The model under review builds one solid part; all positions refer to its coordinate system, in mm. A direction names the side the tool comes from. Coordinates: 2 decimals unless noted, no trailing zeros. Write each loop counter-clockwise with the first axis right and the second up, starting at its lowest first coordinate (ties: lowest second). Pieces come first, ordered by that corner, then holes. Notation, with made-up numbers: (74, 25) -> (127, 25) arc R31 cw to (127, 50) -> close; hole circle Ø10 at (18, 26). An arc over 180 degrees is marked (long way). Write each question's results on one line, items separated by ' | '.
Autodesk Inventor part; units mm, degrees
ref_plane "Work Plane2" through (-3.9, 5.05, 12.4) normal (0, 0, 1) x (1, 0, 0)
ref_plane "Work Plane3" through (-3.9, 5.05, 8) normal (0, 0, 1) x (1, 0, 0)
ref_plane "Work Plane4" through (-13.9917, -57.9, 3) normal (0, 0, 1) x (1, 0, 0)
ref_plane "Work Plane1" through (0, 0, 0) normal (0, 0, 1) x (1, 0, 0)
sketch "Sketch1" plane through (0, 0, 0) normal (0, 0, 1) x (1, 0, 0)
  circle A0 centre (0, -8.95) radius 4.2
  circle A1 centre (0, 8.95) radius 4.2
  circle A2 centre (0, 0) radius 1.4
  circle A3 centre (3.9, 0) radius 0.1
  line L0 (8.9, 16.9) -> (7.9, 17.9)
  line L1 (7.9, 17.9) -> (-7.9, 17.9)
  line L2 (-7.9, 17.9) -> (-8.9, 16.9)
  line L3 (-8.9, 16.9) -> (-8.9, -16.9)
  line L4 (-8.9, -16.9) -> (-7.9, -17.9)
  line L5 (-7.9, -17.9) -> (7.9, -17.9)
  line L6 (7.9, -17.9) -> (8.9, -16.9)
  line L7 (8.9, -16.9) -> (8.9, 16.9)
  point P0 (0, 0)
ref_plane "Work Plane2" through (-3.9, 5.05, 12.4) normal (0, 0, 1) x (1, 0, 0)
ref_plane "Work Plane3" through (-3.9, 5.05, 8) normal (0, 0, 1) x (1, 0, 0)
extrude "Extrusion1" add sketch "Sketch1" along normal up to surface (8 mm away) contours A0 | A1 | L7 L6 L5 L4 L3 L2 L1 L0
sketch "Sketch2" plane through (-7.9, 17.9, 8) normal (0, 0, 1) x (1, 0, 0)
  line L0 (16.8, -1) -> (16.8, -34.8)
  line L1 (15.8, 0) -> (16.8, -1)
  line L2 (0, 0) -> (15.8, 0)
  line L3 (-1, -1) -> (0, 0)
  line L4 (-1, -34.8) -> (-1, -1)
  line L5 (0, -35.8) -> (-1, -34.8)
  line L6 (15.8, -35.8) -> (0, -35.8)
  line L7 (16.8, -34.8) -> (15.8, -35.8)
  circle A0 centre (11.8, -17.9) radius 0.1
  circle A1 centre (7.9, -17.9) radius 1.4
  point P0 (7.9, -17.9)
  point P1 (13.4, -17.9)
  point P2 (2.4, -17.9)
  dimension "d2" = 5.5
  dimension "d3" = 5.5
hole "Hole1" at (5.5, 0, 8) at (-5.5, 0, 8) direction (0, 0, -1) diameter 2.9 end through all counterbore diameter 6 counterbore depth 3.5
sketch "Sketch3" plane through (0, 0, 0) normal (0, 0, -1) x (-1, 0, 0)
  circle A0 centre (0, 8.95) radius 3.9 construction
  circle A1 centre (0, -8.95) radius 3.9 construction
  circle A2 centre (0, 8.95) radius 3.375
  circle A3 centre (0, -8.95) radius 3.375
  point P0 (0, 0)
  dimension "d11" = 6.75
  dimension "d12" = 6.75
extrude "Extrusion2" cut sketch "Sketch3" against normal blind 10
sketch "Sketch4" plane through (0, 0, 0) normal (0, 0, -1) x (-1, 0, 0)
  circle A0 centre (0, 8.95) radius 3.375
  circle A1 centre (0, -8.95) radius 3.375
  circle A2 centre (0, 8.95) radius 3.9
  circle A3 centre (0, -8.95) radius 3.9
  point P0 (0, 0)
  dimension "d15" = 7.8
  dimension "d16" = 7.8
extrude "Extrusion3" cut sketch "Sketch4" against normal blind 4
sketch "Sketch5" plane through (0, 0, 0) normal (0, 0, -1) x (-1, 0, 0)
  circle A0 centre (0, 8.95) radius 3.9
  circle A1 centre (0, 8.95) radius 3.9
  circle A2 centre (0, -8.95) radius 3.9
  circle A3 centre (-5.5, 0) radius 1.45
  circle A4 centre (5.5, 0) radius 1.45
  circle A5 centre (-3.9, 0) radius 0.1
  line L0 (-8.9, 16.9) -> (-7.9, 17.9)
  line L1 (-8.9, -16.9) -> (-8.9, 16.9)
  line L2 (-7.9, -17.9) -> (-8.9, -16.9)
  line L3 (7.9, -17.9) -> (-7.9, -17.9)
  line L4 (8.9, -16.9) -> (7.9, -17.9)
  line L5 (8.9, 16.9) -> (8.9, -16.9)
  line L6 (7.9, 17.9) -> (8.9, 16.9)
  line L7 (-7.9, 17.9) -> (7.9, 17.9)
  line L8 (7.4, -16.2787) -> (7.2787, -16.4)
  line L9 (7.2787, -16.4) -> (-7.2787, -16.4)
  line L10 (-7.2787, -16.4) -> (-7.4, -16.2787)
  line L11 (-7.4, -16.2787) -> (-7.4, 16.2787)
  line L12 (-7.4, 16.2787) -> (-7.2787, 16.4)
  line L13 (-7.2787, 16.4) -> (7.2787, 16.4)
  line L14 (7.2787, 16.4) -> (7.4, 16.2787)
  line L15 (7.4, 16.2787) -> (7.4, -16.2787)
  point P0 (0, 0)
  dimension "d19" = 1.5
extrude "Extrusion4" cut sketch "Sketch5" against normal blind 3 contours A0 | A2 | A3 | A4 | L8 L9 L10 L11 L12 L13 L14 L15
ref_plane "Work Plane4" through (-13.9917, -57.9, 3) normal (0, 0, 1) x (1, 0, 0)
sketch "Sketch6" plane through (-7.9, 17.9, 8) normal (0, 0, 1) x (1, 0, 0)
  circle A0 centre (7.9, -8.95) radius 3.375
  circle A1 centre (7.9, -26.85) radius 3.375
  circle A2 centre (2.4, -17.9) radius 3
  circle A3 centre (13.4, -17.9) radius 3
  line L0 (16.8, -1) -> (16.8, -34.8)
  line L1 (15.8, 0) -> (16.8, -1)
  line L2 (0, 0) -> (15.8, 0)
  line L3 (-1, -1) -> (0, 0)
  line L4 (-1, -34.8) -> (-1, -1)
  line L5 (0, -35.8) -> (-1, -34.8)
  line L6 (15.8, -35.8) -> (0, -35.8)
  line L7 (16.8, -34.8) -> (15.8, -35.8)
  line L8 (16.8, -34.8) -> (16.8, -1)
  line L9 (-1, 0) -> (16.8, 0)
  line L10 (16.8, 0) -> (16.8, -3)
  line L11 (16.8, -3) -> (-1, -3)
  line L12 (-1, -3) -> (-1, 0)
  line L13 (-1, -35.8) -> (16.8, -35.8)
  line L14 (16.8, -35.8) -> (16.8, -32.8)
  line L15 (16.8, -32.8) -> (-1, -32.8)
  line L16 (-1, -32.8) -> (-1, -35.8)
  point P0 (7.9, -17.9)
  dimension "d22" = 3
  dimension "d23" = 3
extrude "Extrusion5" cut sketch "Sketch6" against normal up to surface (5 mm away) contours L0 L11 L4 L3 L2 L1 | L1 L9 L10 | L0 L7 L6 L5 L4 L15 | L3 L12 L9 | L14 L13 L7 | L5 L13 L16
sketch "Sketch7" plane through (0, 0, 0) normal (0, 0, -1) x (-1, 0, 0)
  line L0 (7.4, 16.2787) -> (7.4, -16.2787)
  line L1 (7.4, -16.2787) -> (7.2787, -16.4)
  line L2 (7.2787, -16.4) -> (-7.2787, -16.4)
  line L3 (-7.2787, -16.4) -> (-7.4, -16.2787)
  line L4 (-7.4, -16.2787) -> (-7.4, 16.2787)
  line L5 (-7.4, 16.2787) -> (-7.2787, 16.4)
  line L6 (-7.2787, 16.4) -> (7.2787, 16.4)
  line L7 (7.2787, 16.4) -> (7.4, 16.2787)
  line L8 (-8.9, 16.9) -> (-7.9, 17.9)
  line L9 (-8.9, -16.9) -> (-8.9, 16.9)
  line L10 (-7.9, -17.9) -> (-8.9, -16.9)
  line L11 (7.9, -17.9) -> (-7.9, -17.9)
  line L12 (8.9, -16.9) -> (7.9, -17.9)
  line L13 (8.9, 16.9) -> (8.9, -16.9)
  line L14 (7.9, 17.9) -> (8.9, 16.9)
  line L15 (-7.9, 17.9) -> (7.9, 17.9)
  line L16 (7.4, 14.9) -> (7.4, -14.9)
  line L17 (7.4, 13.4) -> (-7.4, 13.4)
  line L18 (-7.4, 13.4) -> (-7.4, 16.4)
  line L19 (-7.4, 16.4) -> (7.4, 16.4)
  line L20 (7.4, 16.4) -> (7.4, 13.4)
  line L21 (7.4, -13.4) -> (-7.4, -13.4)
  line L22 (-7.4, -13.4) -> (-7.4, -16.4)
  line L23 (-7.4, -16.4) -> (7.4, -16.4)
  line L24 (7.4, -16.4) -> (7.4, -13.4)
  point P0 (0, 0)
  dimension "d26" = 3
  dimension "d27" = 3
extrude "Extrusion6" add sketch "Sketch7" against normal up to surface (3 mm away) contours L0 L17 L4 L5 L6 L7 | L5 L18 L19 | L0 L1 L2 L3 L4 L21 | L24 L23 L1 | L3 L23 L22
sketch "Sketch8" plane through (0, 0, 0) normal (0, 0, -1) x (-1, 0, 0)
  line L0 (7.4, 13.4) -> (-7.4, 13.4)
  line L1 (-7.4, -13.4) -> (-7.4, 13.4)
  line L2 (-7.4, -13.4) -> (7.4, -13.4)
  line L3 (7.4, 13.4) -> (7.4, -13.4)
  circle A0 centre (0, 8.95) radius 3.9
  circle A1 centre (0, -8.95) radius 3.9
  circle A2 centre (-5.5, 0) radius 1.45
  circle A3 centre (5.5, 0) radius 1.45
  circle A4 centre (0, 0) radius 1.4
  circle A5 centre (-3.9, 0) radius 0.1
  point P0 (0, 0)
extrude "Extrusion7" add sketch "Sketch8" against normal up to surface (3 mm away)
properties part number "Omnivision_Objectivelens_mount"
Q1. Draft analysis for pull direction Y (two halves, no side actions). For faces 1 (the flat face through (2, 12, 4)), 2 (the flat face through (-8.4, 17.4, 1.5)), 3 (the flat face through (0, -14.9, 6)), state which applies: pulls with the +Y half, pulls with the -Y half, needs draft (parallel to the pull), parting line crosses it, or undercut.
Solution:
face 1: undercut | face 2: pulls with the +Y half | face 3: pulls with the -Y half
Q2. Machinability: for faces 4 (the cylindrical face through (0.845, 5.143, 1.972)), 5 (the flat face through (0, -17.9, 1)), 6 (the flat face through (0, -16, 3)), 7 (the cylindrical face through (-2.57, 0.65, 6.23)), which of the approach directions +Z, -Z, +X, -X, +Y, -Y give a long, thin tool a straight path to every point of the face, cutting with its end or side? Answer none if there is none.
Solution:
face 4: -Z | face 5: +Z, -Z, +X, -X, -Y | face 6: +Z, +X, -X, -Y | face 7: +Z
Q3. Add section C-C (z = 1.75). Write out the cut boundary in (x, y), plus the area to 3 significant figures.
Solution:
outline: (-8.9, -16.9) -> (-7.9, -17.9) -> (7.9, -17.9) -> (8.9, -16.9) -> (8.9, 16.9) -> (7.9, 17.9) -> (-7.9, 17.9) -> (-8.9, 16.9) -> close; hole circle Ø2.9 at (-5.5, 0); hole circle Ø7.8 at (0, -8.95); hole circle Ø7.8 at (0, 8.95); hole circle Ø2.8 at (0, 0); hole circle Ø0.2 at (3.9, 0); hole circle Ø2.9 at (5.5, 0) | area: 520 mm²
Q4. Clearance check with flat-ended pins moving along their axes: P1, Ø1.5, axis at x = 2, y = 16, coming from the +Z side; P2, Ø3, axis at x = -6, y = -0.5, coming from the +Z side. State where each tip first meets the part, or that it passes through.
Solution:
P1: z = 3 | P2: z = 4.5
Q5. For line 1 (Y direction, x = 0, z = 2.2); line 2 (Y direction, x = 0, z = 5.5) (3 decimals); line 3 (X direction, y = 0, z = 7.1), list the stretches that pass through material, from the lowest coordinate up. Write a range as from..to.
Solution:
line 1: -17.9..-12.85, -5.05..-1.4, 1.4..5.05, 12.85..17.9 | line 2: -14.9..-12.325, -5.575..-1.4, 1.4..5.575, 12.325..14.9 | line 3: -8.9..-8.5, -2.5..-1.4, 1.4..2.5, 8.5..8.9
Q6. Add section B-B (x = 0). Write out the cut boundary in (y, z) (3 decimals), plus the area to 3 significant figures.
Solution:
outline: (-17.9, 0) -> (-12.85, 0) -> (-12.85, 4) -> (-12.325, 4) -> (-12.325, 8) -> (-14.9, 8) -> (-14.9, 3) -> (-17.9, 3) -> close; (-5.575, 4) -> (-5.05, 4) -> (-5.05, 0) -> (-1.4, 0) -> (-1.4, 8) -> (-5.575, 8) -> close; (1.4, 0) -> (5.05, 0) -> (5.05, 4) -> (5.575, 4) -> (5.575, 8) -> (1.4, 8) -> close; (12.325, 4) -> (12.85, 4) -> (12.85, 0) -> (17.9, 0) -> (17.9, 3) -> (14.9, 3) -> (14.9, 8) -> (12.325, 8) -> close | area: 118 mm²
Q7. Add section D-D (y = 6). Write out the cut boundary in (x, z), plus the area to 3 significant figures.
Solution:
outline: (-8.9, 0) -> (-2.55, 0) -> (-2.55, 4) -> (-1.64, 4) -> (-1.64, 8) -> (-8.9, 8) -> close; (1.64, 4) -> (2.55, 4) -> (2.55, 0) -> (8.9, 0) -> (8.9, 8) -> (1.64, 8) -> close | area: 109 mm²
Q8. Add section A-A (z = 6.75). Write out the cut boundary in (x, y) (3 decimals), plus the area to 3 significant figures.
Solution:
outline: (-8.9, -14.9) -> (8.9, -14.9) -> (8.9, 14.9) -> (-8.9, 14.9) -> close; hole circle Ø6 at (-5.5, 0); hole circle Ø6.75 at (0, -8.95); hole circle Ø6.75 at (0, 8.95); hole circle Ø2.8 at (0, 0); hole circle Ø6 at (5.5, 0) | area: 396 mm²
